Check sheet for the modelled part. Datum: model origin and axes. Units: mm. A direction names the side the tool comes from. Give positions to 0.01 mm unless a question says otherwise; leave off trailing zeros. Order: outer loops, then holes, each group sorted by start corner. A loop starts at its lowest first (then second) coordinate and runs counter-clockwise, first axis right, second up. Notation, with made-up numbers: M -25.5,80 L 21.5,80 A26 ccw 21.5,100 Z; hole C 29,57.5 d4. An arc over 180 degrees is marked long. Answer in a Markdown table with one row per item. Add a question column.
Autodesk Inventor part; units mm, degrees
ref_plane "YZ Plane" through (0, 0, 0) normal (1, 0, 0) x (0, 1, 0)
ref_plane "XZ Plane" through (0, 0, 0) normal (0, 1, 0) x (-1, 0, 0)
ref_plane "XY Plane" through (0, 0, 0) normal (0, 0, 1) x (1, 0, 0)
sketch "草图1" plane through (0, 0, 0) normal (0, 0, 1) x (1, 0, 0)
  line L0 (0, 0) -> (0, 17.5565)
  line L1 (-20, 2.5) -> (20, 2.5)
  line L2 (20, 2.5) -> (20, -2.5)
  line L3 (-20, -2.5) -> (-20, 2.5)
  line L4 (-20, 2.5) -> (20, -2.5) construction
  line L5 (20, 2.5) -> (-20, -2.5) construction
  line L6 (0, -7.5) -> (14, -7.5)
  line L7 (0, -7.5) -> (-14, -7.5)
  line L8 (-10.5, -2.5) -> (-14, -7.5)
  line L9 (14, -7.5) -> (10.5, -2.5)
  line L10 (20, -2.5) -> (10.5, -2.5)
  line L11 (-10.5, -2.5) -> (-20, -2.5)
  dimension "d1" = 40
  dimension "d2" = 5
  dimension "d5" = 14
  dimension "d8" = 21
extrude "拉伸1" add sketch "草图1" along normal blind 50
sketch "草图2" plane through (0, 0, 0) normal (0, 0, -1) x (-1, 0, 0)
  line L0 (-20, 2.5) -> (20, 2.5)
  line L1 (0, 2.5) -> (0, 17.5)
  arc A0 (-12, 17.5) -> (12, 17.5) centre (0, 17.5) ccw
  line L2 (-12, 17.5) -> (-12, 2.5)
  line L3 (12, 17.5) -> (12, 2.5)
  point P0 (0, 0)
  dimension "d11" = 15
  dimension "d12" = 24
extrude "拉伸2" add sketch "草图2" against normal blind 10
sketch "草图3" plane through (-20, 2.5, 50) normal (0, 1, 0) x (1, 0, 0)
  line L0 (40, 0) -> (0, 0)
  line L1 (20, 0) -> (20, 18)
  circle A0 centre (20, 18) radius 4
  point P0 (20, 50)
  dimension "d15" = 18
  dimension "d16" = 8
extrude "拉伸3" cut sketch "草图3" against normal blind 20
properties part number "2-6"
Q1. Cross-section at A-A (z = 32). Record the boundary of the cut face in (x, y).
Q2. Cross-section at B-B (x = 0). Record the boundary of the cut face in (y, z), and give its area (3 significant figures).
Q3. Draft check along X on faces 4 (the flat face through (12, 10, 5)), 5 (the cylindrical face through (-0.521, -2.43, 28.034)), 6 (the flat face through (0, 2.5, 25)). Enter one of: pulls with the +X half, pulls with the -X half, needs draft (parallel to the pull), parting line crosses it, or undercut.
Q4. Go/stop test with flat-tipped pins: pin 1 (10 mm diameter, centred on x = -7, z = 28, fed in from +Y); pin 2 (5 mm diameter, centred on y = 9, z = 3, fed in from -X); pin 3 (3 mm diameter, centred on x = 5.5, y = -4.5, fed in from -Z); pin 4 (3 mm diameter, centred on y = 11.5, z = 7, fed in from +X). Record where each tip stops, or that it passes through.
Q5. Thickness scan on probe 1 along Z at (x, y) = (0, -3.25); probe 2 along Y at (x, z) = (-1, 43); probe 3 along X at (y, z) = (11, 9). Record the ranges inside material, lowest first.
Q6. Tool access check on faces 1 (the flat face through (0, 5, 10)), 2 (the flat face through (-12, 10, 5)), 3 (the flat face through (12.27, -5.03, 24.65)). Record the directions out of +Z, -Z, +X, -X, +Y, -Y that give a thin tool (end or side, any length) a straight path to the whole face; none if there is none.
Q7. Cross-section at C-C (y = -1.5). Record the boundary of the cut face in (x, z), and give its area (3 significant figures).
Q8. Cross-section at D-D (y = 14). Record the boundary of the cut face in (x, z).
Values follow:
| question | item | result |
|---|---|---|
| 1 | outline | M -20,-2.5 L -10.5,-2.5 L -14,-7.5 L -4,-7.5 L -4,2.5 L -20,2.5 Z; M 4,-7.5 L 14,-7.5 L 10.5,-2.5 L 20,-2.5 L 20,2.5 L 4,2.5 Z |
| 2 | outline | M -7.5,0 L 5.5,0 L 5.5,10 L 2.5,10 L 2.5,28 L -7.5,28 Z; M -7.5,36 L 2.5,36 L 2.5,50 L -7.5,50 Z |
| 2 | area | 450 mm² |
| 3 | face 4 | pulls with the +X half |
| 3 | face 5 | undercut |
| 3 | face 6 | needs draft |
| 4 | pin 1 | y = 2.5 |
| 4 | pin 2 | x = -12 |
| 4 | pin 3 | z = 0 |
| 4 | pin 4 | x = 12 |
| 5 | probe 1 | 0 to 28, 36 to 50 |
| 5 | probe 2 | -7.5 to 2.5 |
| 5 | probe 3 | -12 to -10.09, 10.09 to 12 |
| 6 | face 1 | +Z, +X, -X, +Y |
| 6 | face 2 | +Z, -Z, -X, +Y |
| 6 | face 3 | +Z, -Z, +X |
| 7 | outline | M -20,0 L 20,0 L 20,50 L -20,50 Z; hole C 0,32 d8 |
| 7 | area | 1,950 mm² |
| 8 | outline | M -12,0 L -11.48,0 L -11.48,10 L -12,10 Z; M 11.48,0 L 12,0 L 12,10 L 11.48,10 Z |
